from build123d import *

# Parameters (mm, degrees)
F0_W     = 151
F0_H     = 82
F1_DEPTH = 40
F2_W     = 15
F2_H     = 40
F3_DEPTH = 41
F4_W     = 22.5
F4_H     = 30
F5_DEPTH = 50
F6_R     = 1.5
F7_DEPTH = 5


with BuildPart() as f1:
    # F0 (on Top) → F1 (new body)
    with BuildSketch(Plane.XY):
        Rectangle(F0_W, F0_H)
    extrude(amount=F1_DEPTH)

    # F2 (on face) → F3 (cut)
    with BuildSketch(Plane.XY.offset(40)):
        with Locations((-68, 19)):
            Rectangle(F2_W, F2_H)
    extrude(amount=-F3_DEPTH, mode=Mode.SUBTRACT)

    # F4 (on face) → F5 (cut)
    with BuildSketch(Plane(origin=(-75.5, 0, 0), x_dir=(0, -1, 0), z_dir=(-1, 0, 0))):
        with Locations((24.75, 23)):
            Rectangle(F4_W, F4_H)
    extrude(amount=-F5_DEPTH, mode=Mode.SUBTRACT)

    # F6 (on face) → F7 (cut)
    with BuildSketch(Plane.YZ.offset(75.5)):
        with Locations((-25, 29)):
            Circle(F6_R)
        with Locations((28, 29)):
            Circle(F6_R)
    extrude(amount=-F7_DEPTH, mode=Mode.SUBTRACT)


solid = f1.part
Build history of the part. All positions in model axes, mm. A direction names the side the tool comes from. Coordinates: 2 decimals unless noted, no trailing zeros. Order: outer loops, then holes, each group sorted by start corner. A loop starts at its lowest first (then second) coordinate and runs counter-clockwise, first axis right, second up. Notation, with made-up numbers: M 71.5,87 L 117.5,87 A14 ccw 117.5,97 Z; hole C 68.25,39.25 d11. An arc over 180 degrees is marked long. One line per question, with ' | ' between items. Start each with the question number.
Q1. Two-plate mould, pull along Z, no slides. Class faces 4 (the face through (70.5, 28, 29)), 5 (the face through (-1, 1, 0)), 6 (the face through (-68, -1, 20)): +Z half, -Z half, draft (parallel to the pull), parting line (faces both ways), or undercut.
Q2. Saw through at C-C (z = 6.5). List the corners of the cut face in (x, y).
Q3. Saw through at A-A (x = -62). List the corners of the cut face in (y, z), then the cut area to 4 significant figures.
Q4. Saw through at B-B (x = -42.5). List the corners of the cut face in (y, z), then the cut area to 4 significant figures.
Q5. Probe L1, parallel to Y at x = -61, z = 23; L2, parallel to Z at x = 73, y = -25; L3, parallel to Y at x = -38, z = 37. List the from-to ranges inside material, lowest first. Write a range as from..to.
Q6. 3-axis set-ups, long thin cutter, end or side, ignore diameter. For faces 1 (the face through (-51, -25, 8)), 2 (the face through (-68, 39, 20)), 3 (the face through (73.04, -26.11, 30.01)): which of +Z, -Z, +X, -X, +Y, -Y reach the whole face in a straight line?
Q7. Flat gauge pins, fed straight in: pin 1 Ø1.8 at (y, z) = (28, 29) entering from -X; pin 2 Ø18 at (x, y) = (-46, -20) entering from -Z; pin 3 Ø0.9 at (y, z) = (28, 29) entering from +X. Where does each tip first touch, or does it go through?
Q8. Saw through at D-D (y = -25). List the corners of the cut face in (x, z).
Check values:
1) face 4: undercut | face 5: -Z half | face 6: draft
2) outline: M -75.5,-41 L 75.5,-41 L 75.5,41 L -75.5,41 L -75.5,39 L -60.5,39 L -60.5,-1 L -75.5,-1 Z
3) outline: M -41,0 L -1,0 L -1,40 L -41,40 Z; M 39,0 L 41,0 L 41,40 L 39,40 Z; hole M -36,8 L -13.5,8 L -13.5,38 L -36,38 Z | area: 1,005 mm2
4) outline: M -41,0 L 41,0 L 41,40 L -41,40 Z; hole M -36,8 L -13.5,8 L -13.5,38 L -36,38 Z | area: 2,605 mm2
5) L1: y = -41..-36, -13.5..-1, 39..41 | L2: z = 0..27.5, 30.5..40 | L3: y = -41..-36, -13.5..41
6) face 1: -X | face 2: +Z, -Z, -X | face 3: +X
7) pin 1: stops at x = -60.5 | pin 2: stops at z = 0 | pin 3: stops at x = 70.5
8) outline: M -75.5,0 L 75.5,0 L 75.5,27.5 L 70.5,27.5 L 70.5,30.5 L 75.5,30.5 L 75.5,40 L -75.5,40 L -75.5,38 L -25.5,38 L -25.5,8 L -75.5,8 Z
